Could you check a few things on this drawing? It's one solid part, dimensions in mm from its lowest x, y, z. A direction names the side the tool comes from. Coordinates: 2 decimals unless noted, no trailing zeros. Order: outer loops, then holes, each group sorted by start corner. A loop starts at its lowest first (then second) coordinate and runs counter-clockwise, first axis right, second up. Notation, with made-up numbers: (59.25, 82.5) - (116.25, 82.5) arc R21 ccw to (116.25, 116.5) - close; hole circle Ø6 at (-2.5, 48.5). An arc over 180 degrees is marked (long way). Return JSON: item names as keys, results as strings. Group by question number.
1) Imagine slicing it at D-D (z = 1). Write out the boundary of the cut face in (x, y).
2) If I drill on line 1 along X through (y, z) = (10, 7.5); line 2 along X through (y, z) = (20.25, 7.5); line 3 along Z through (x, y) = (16.75, 14.25), over which ranges is the centre line in solid material (lowest first)?
3) Imagine slicing it at B-B (x = 16.75). Write out the boundary of the cut face in (y, z).
4) Imagine slicing it at C-C (y = 23). Write out the boundary of the cut face in (x, z).
5) Imagine slicing it at A-A (y = 12.25). Write out the boundary of the cut face in (x, z).
6) For pin 1 Ø4.5 at (x, z) = (17, 9.5) entering from -Y; pin 2 Ø8 at (x, z) = (16.75, 7.5) entering from +Y; pin 3 Ø5 at (x, z) = (26, 4.5) entering from -Y, each with a flat end and sliding along its axis, tell me the tip position at first contact or that it passes through.
7) Which directions (+Z, -Z, +X, -X, +Y, -Y) give clear straight access to the entire face, cutting with the end or side of a thin tool? Please do the marked faces 1, 2 and 3.
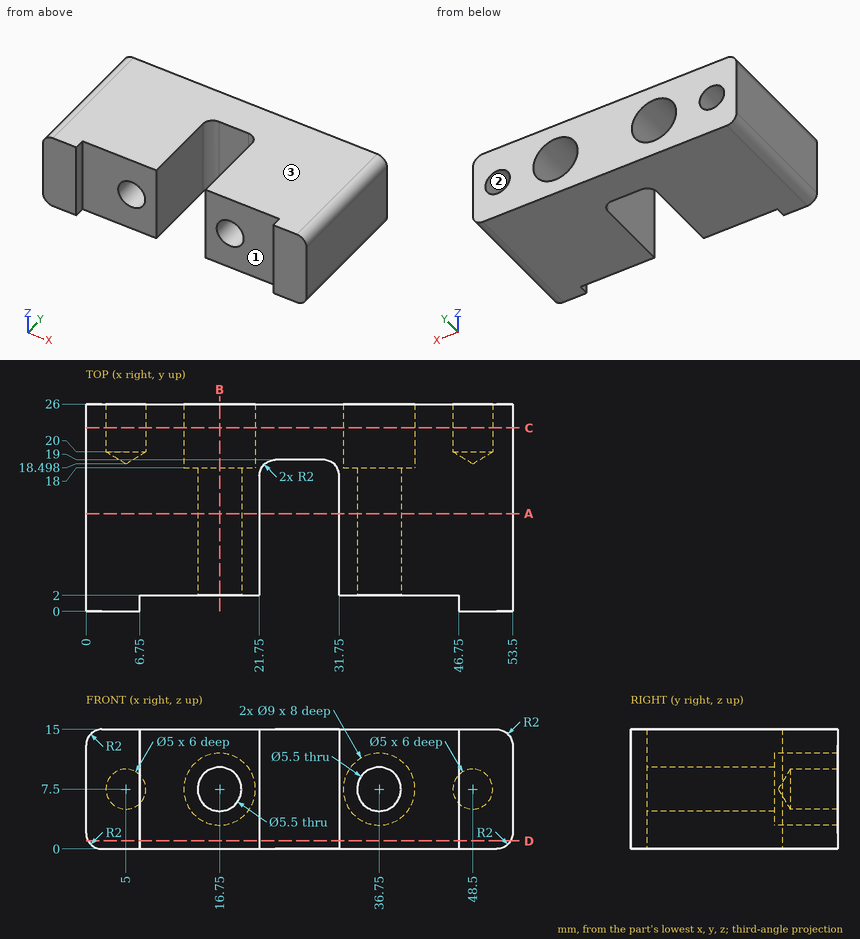
Calculated:
{
 "1": {"outline": "(0.27, 0) - (6.75, 0) - (6.75, 2) - (21.75, 2) - (21.75, 17) arc R2 cw to (23.75, 19) - (29.75, 19) arc R2 cw to (31.75, 17) - (31.75, 2) - (46.75, 2) - (46.75, 0) - (53.23, 0) - (53.23, 26) - (0.27, 26) - close"},
 "2": {"line 1": "0 to 14, 19.5 to 21.75, 31.75 to 34, 39.5 to 53.5", "line 2": "0 to 2.5, 7.5 to 12.25, 21.25 to 32.25, 41.25 to 46, 51 to 53.5", "line 3": "0 to 4.75, 10.25 to 15"},
 "3": {"outline": "(2, 0) - (26, 0) - (26, 3) - (18, 3) - (18, 4.75) - (2, 4.75) - close; (2, 10.25) - (18, 10.25) - (18, 12) - (26, 12) - (26, 15) - (2, 15) - close"},
 "4": {"outline": "(0, 2) arc R2 ccw to (2, 0) - (51.5, 0) arc R2 ccw to (53.5, 2) - (53.5, 13) arc R2 ccw to (51.5, 15) - (2, 15) arc R2 ccw to (0, 13) - close; hole circle Ø5 at (5, 7.5); hole circle Ø9 at (16.75, 7.5); hole circle Ø9 at (36.75, 7.5); hole circle Ø5 at (48.5, 7.5)"},
 "5": {"outline": "(0, 2) arc R2 ccw to (2, 0) - (21.75, 0) - (21.75, 15) - (2, 15) arc R2 ccw to (0, 13) - close; (31.75, 0) - (51.5, 0) arc R2 ccw to (53.5, 2) - (53.5, 13) arc R2 ccw to (51.5, 15) - (31.75, 15) - close; hole circle Ø5.5 at (16.75, 7.5); hole circle Ø5.5 at (36.75, 7.5)"},
 "6": {"pin 1": "y = 2", "pin 2": "y = 18", "pin 3": "y = 18.98"},
 "7": {"face 1": "+Z, -Z, -Y", "face 2": "+Y", "face 3": "+Z, +X, -X, +Y, -Y"}
}
